Could you check a few things on this model? Use its own coordinates, in mm. Face numbers are marked on the shaded views. A direction names the side the tool comes from. Give positions to 0.01 mm unless a question says otherwise; leave off trailing zeros. Write each loop counter-clockwise with the first axis right and the second up, starting at its lowest first coordinate (ties: lowest second). Pieces come first, ordered by that corner, then holes. Notation, with made-up numbers: (-32, -15) -> (-5, -15) arc R33 ccw to (-5, 18) -> close; hole circle Ø5 at (-27.5, 49.5). An arc over 180 degrees is marked (long way). One line per question, with ' | ' between items.
from build123d import *

# Parameters (mm, degrees)
SKETCH_1_R          = 1.6
EXTRUDE_1_DEPTH     = 25
SKETCH_2_W          = 2.45
SKETCH_2_H          = 19.896013553
EXTRUDE_2_DEPTH     = 40
SKETCH_3_R          = 1.5
CUT_EXTRUDE_1_DEPTH = 90.582364336
SKETCH_4_W          = 40
SKETCH_4_H          = 4
EXTRUDE_3_DEPTH     = 25
FILLET_4_R          = 10
FILLET_5_R          = 10


with BuildPart() as part:
    # 草图1 → 凸台-拉伸1 (new body)
    # profile 1 of 2: a face of its own
    with BuildSketch(Plane(origin=(0, 0, 0), x_dir=(0, 0, -1), z_dir=(1, 0, 0))):
        with BuildLine():
            ThreePointArc((-47.85, 0), (-46.25, 1.6), (-44.65, 0))
            Line((-44.65, 0), (-42.5, 0))
            ThreePointArc((-42.5, 0), (-16.298006013, 39.25079617), (30, 30.103986447))
            Line((30, 30.103986447), (30, 50))
            Line((30, 50), (0, 50))
            ThreePointArc((0, 50), (-35.355339059, 35.355339059), (-50, 0))
            Line((-50, 0), (-47.85, 0))
        make_face()
        with Locations((-23.125, 40.053674925)):
            Circle(SKETCH_1_R, mode=Mode.SUBTRACT)
        with Locations((23.125, 40.053674925)):
            Circle(SKETCH_1_R, mode=Mode.SUBTRACT)
    # profile 2 of 2: a face of its own
    with BuildSketch(Plane(origin=(0, 0, 0), x_dir=(0, 0, -1), z_dir=(1, 0, 0))):
        with BuildLine():
            Line((-42.5, 0), (-44.65, 0))
            ThreePointArc((-44.65, 0), (-46.25, -1.6), (-47.85, 0))
            Line((-47.85, 0), (-50, 0))
            ThreePointArc((-50, 0), (-35.355339059, -35.355339059), (0, -50))
            Line((0, -50), (30, -50))
            Line((30, -50), (30, -30.103986447))
            ThreePointArc((30, -30.103986447), (-16.298006013, -39.25079617), (-42.5, 0))
        make_face()
        with Locations((-23.125, -40.053674925)):
            Circle(SKETCH_1_R, mode=Mode.SUBTRACT)
        with Locations((23.125, -40.053674925)):
            Circle(SKETCH_1_R, mode=Mode.SUBTRACT)
    extrude(amount=EXTRUDE_1_DEPTH)

    # 草图2 → 凸台-拉伸2 (add)
    with BuildSketch(Plane(origin=(0, 0, -30), x_dir=(-1, 0, 0), z_dir=(0, 0, -1))):
        with Locations((-23.775, 40.051993223)):
            Rectangle(SKETCH_2_W, SKETCH_2_H)
        with Locations((-1.225, 40.051993223)):
            Rectangle(SKETCH_2_W, SKETCH_2_H)
        with Locations((-1.225, -40.051993223)):
            Rectangle(SKETCH_2_W, SKETCH_2_H)
        with Locations((-23.775, -40.051993223)):
            Rectangle(SKETCH_2_W, SKETCH_2_H)
    extrude(amount=EXTRUDE_2_DEPTH)

    # 草图3 → 切除-拉伸1 (cut, through all)
    with BuildSketch(Plane(origin=(25, 0, 0), x_dir=(0, 0, -1), z_dir=(1, 0, 0))):
        with Locations((60, -40.051993223)):
            Circle(SKETCH_3_R)
        with Locations((40, -40.051993223)):
            Circle(SKETCH_3_R)
        with Locations(Location((40.013969679, 40.055824631, 0), (0, 0, 270))):
            Circle(SKETCH_3_R)
        with Locations(Location((60.013968462, 40.048849193, 0), (0, 0, 270))):
            Circle(SKETCH_3_R)
    extrude(amount=-CUT_EXTRUDE_1_DEPTH, mode=Mode.SUBTRACT)

    # 草图4 → 凸台-拉伸3 (add)
    with BuildSketch(Plane(origin=(25, 0, 0), x_dir=(0, 0, -1), z_dir=(1, 0, 0))):
        with Locations((20, 52)):
            Rectangle(SKETCH_4_W, SKETCH_4_H)
        with Locations((20, -52)):
            Rectangle(SKETCH_4_W, SKETCH_4_H)
    extrude(amount=-EXTRUDE_3_DEPTH)

    # 圆角4
    # the kernel refuses this fillet: 10 mm, written as the material it takes off along each edge
    with BuildSketch(Plane(origin=(45, -54, 0), x_dir=(0, 0, -1), z_dir=(-1, 0, 0))) as fillet_4_piece_1:
        with BuildLine():
            CenterArc((8, -10), FILLET_4_R, 90, 53.130102354)
            Line((0, -4), (-0.16, -3.88))
            ThreePointArc((-0.16, -3.88), (-0.2, -2), (-0.2, 0))
            Line((-0.2, 0), (0, 0.2))
            Line((0, 0.2), (8, 0.2))
            Line((8, 0.2), (8, 0))
        make_face()
    extrude(amount=65, mode=Mode.SUBTRACT)
    with BuildSketch(Plane(origin=(45, 54, 0), x_dir=(0, 0, -1), z_dir=(-1, 0, 0))) as fillet_4_piece_2:
        with BuildLine():
            CenterArc((8, 10), FILLET_4_R, 216.869897646, 53.130102354)
            Line((0, 4), (-0.16, 3.88))
            ThreePointArc((-0.16, 3.88), (-0.2, 2), (-0.2, 0))
            Line((-0.2, 0), (0, -0.2))
            Line((0, -0.2), (8, -0.2))
            Line((8, -0.2), (8, 0))
        make_face()
    extrude(amount=65, mode=Mode.SUBTRACT)

    # 圆角5
    fillet_5_edges = [part.edges().sort_by_distance(p)[0] for p in [
        (12.5, -50, 0),
        (12.5, 50, 0),
    ]]
    fillet(fillet_5_edges, radius=FILLET_5_R)


solid = part.part
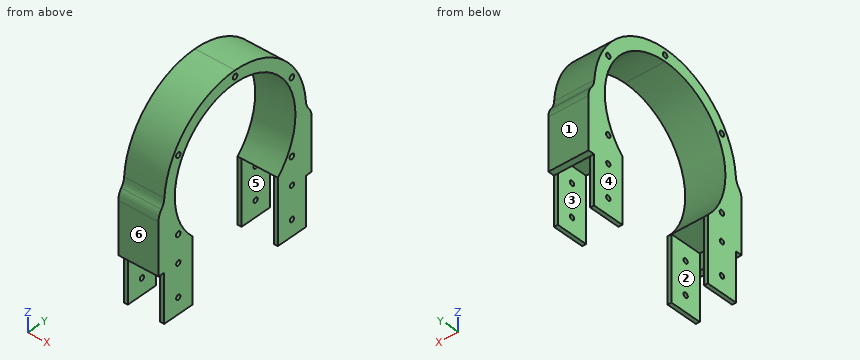
Q1. Will these pins go through, and if not, where does the flat tip stop? pin 1 (2 mm diameter, centred on x = 17, y = -28.5, fed in from +Z); pin 2 (3 mm diameter, centred on x = 15.5, y = 52.5, fed in from -Z); pin 3 (5 mm diameter, centred on x = 17.5, y = -25.5, fed in from -Z).
Answer below:
pin 1: stops at z = 41.76 | pin 2: stops at z = -40 | pin 3: stops at z = 31.97
Q2. Imagine slicing it at C-C on z = 23. Please give me the cut outline in (x, y), and give its area (3 significant figures).
Answer below:
outline: (0, -44.4) -> (25, -44.4) -> (25, -41.65) -> (0, -41.65) -> close; (0, -38.46) -> (25, -38.46) -> (25, -35.74) -> (0, -35.74) -> close; (0, 35.74) -> (25, 35.74) -> (25, 38.46) -> (0, 38.46) -> close; (0, 41.65) -> (25, 41.65) -> (25, 44.4) -> (0, 44.4) -> close | area: 273 mm^2
Q3. Imagine slicing it at D-D on x = 11.25. Count the separate pieces of the cut face and the enclosed holes in it, and give its area (3 significant figures).
Answer below:
separate pieces: 1 | enclosed holes: 5 | area: 2,030 mm^2
Q4. If I drill on line 1 along X through (y, z) = (-46, -39); line 2 along Y through (x, z) = (19, 24.5); line 3 along Y through (x, z) = (1.5, -40.5), over which ranges is the centre line in solid material (lowest first)?
Answer below:
line 1: x = 0 to 2.45, 22.55 to 25 | line 2: y = -43.59 to -40.87, -39.24 to -34.73, 34.73 to 39.24, 40.87 to 43.59 | line 3: y = -50 to -41.47, -38.64 to -30.1, 30.1 to 38.64, 41.47 to 50
Q5. On a 3-axis mill with a long thin cutter (end or side, diameter ignored), from which of +Z, -Z, +X, -X, +Y, -Y can I reach the whole of each face in a straight line? I mean the marked faces 1 and 2. Say none if no direction works.
Answer below:
face 1: +Z, -Z, +X, -X, +Y | face 2: -Z
Q6. Imagine slicing it at A-A on z = -33. Please give me the cut outline in (x, y).
Answer below:
outline: (0, -54) -> (25, -54) -> (25, -30.1) -> (22.55, -30.1) -> (22.55, -50) -> (2.45, -50) -> (2.45, -30.1) -> (0, -30.1) -> close; (0, 30.1) -> (2.45, 30.1) -> (2.45, 50) -> (22.55, 50) -> (22.55, 30.1) -> (25, 30.1) -> (25, 54) -> (0, 54) -> close
Q7. If we mould it in two halves opening along Y, with no side actions, what happens to the marked faces 3, 4, 5 and 6? For each: +Y half, -Y half, draft (parallel to the pull), parting line (faces both ways), or undercut.
Answer below:
face 3: undercut | face 4: draft | face 5: undercut | face 6: -Y half
Q8. Imagine slicing it at B-B on y = -34.5. Please give me the cut outline in (x, z).
Answer below:
outline: (0, -70) -> (2.45, -70) -> (2.45, -30) -> (22.55, -30) -> (22.55, -70) -> (25, -70) -> (25, -24.82) -> (0, -24.82) -> close; (0, 24.82) -> (25, 24.82) -> (25, 36.19) -> (0, 36.19) -> close
